from build123d import *

# Parameters (mm, degrees)
F0_R     = 50
F0_W     = 40
F0_H     = 40
F1_DEPTH = 25
F2_R     = 5
F3_SIZE2 = 5
F3_SIZE  = 2.3315382908


with BuildPart() as f1:
    # F0 (on Top) → F1 (new body)
    with BuildSketch(Plane.XY):
        Circle(F0_R)
        with Locations((0, -3.4369069617)):
            Rectangle(F0_W, F0_H, mode=Mode.SUBTRACT)
    extrude(amount=F1_DEPTH)

    # F2
    f2_edges = [f1.edges().sort_by_distance(p)[0] for p in [
        (0, 16.563093, 25),
        (-20, -3.436907, 25),
        (20, -3.436907, 25),
        (0, -23.436907, 25),
    ]]
    fillet(f2_edges, radius=F2_R)

    # F3
    f3_edges = [f1.edges().sort_by_distance(p)[0] for p in [
        (0, -23.436907, 0),
        (-20, -3.436907, 0),
        (0, 16.563093, 0),
        (20, -3.436907, 0),
    ]]
    f3_side = f1.faces().sort_by_distance((-48.585786, 0, 0))[0]
    chamfer(f3_edges, length=F3_SIZE, length2=F3_SIZE2, reference=f3_side)


solid = f1.part
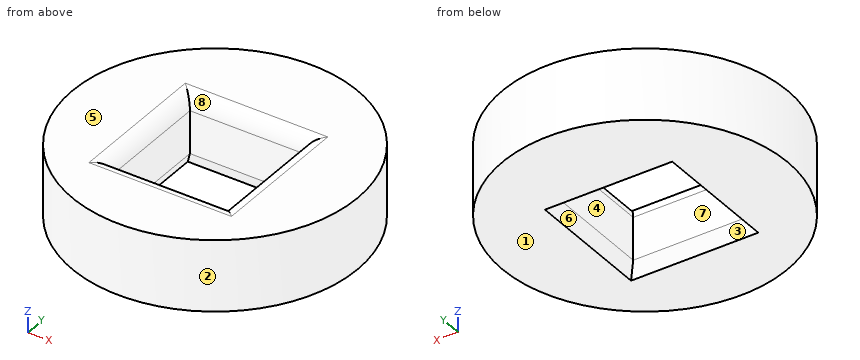
Design review of the part built by this model. Coordinates are the model's own, in mm. Face numbers are marked on the shaded views. A direction names the side the tool comes from. Round coordinates to 2 decimals unless told otherwise and drop trailing zeros. Loops run counter-clockwise (first coordinate to the right, second up) from the corner with the lowest first, then second, coordinate; pieces in that order, holes last. Notation, with made-up numbers: (56.5, 9) - (83.5, 9) arc R10 cw to (83.5, 14) - close; hole circle Ø10 at (52.5, -22). An arc over 180 degrees is marked (long way). One line per question, with ' | ' between items.
1. We need section A-A, the plane x = 0. State the section outline as (y, z) points, and give its area (3 significant figures).
Results are:
outline: (-50, 0) - (-25.77, 0) - (-23.44, 5) - (-23.44, 20) arc R5 ccw to (-28.44, 25) - (-50, 25) - close; (16.56, 5) - (18.89, 0) - (50, 0) - (50, 25) - (21.56, 25) arc R5 ccw to (16.56, 20) - close | area: 1,480 mm²
2. For L1, parallel to Y at x = -10, z = 15; L2, parallel to X at y = -1.5, z = 8.5; L3, parallel to Y at x = 2, z = 16.75, list the stretches that pass through material, from the lowest coordinate up. Write a range as [from, to].
Results are:
L1: y = [-48.99, -23.44], [16.56, 48.99] | L2: x = [-49.98, -20], [20, 49.98] | L3: y = [-49.96, -23.44], [16.56, 49.96]
3. Clearance check with flat-ended pins moving along their axes: P1, Ø1.5, axis at x = 30, z = 17.5, coming from the -Y side; P2, Ø7.5, axis at y = -9, z = 13.5, coming from the -X side; P3, Ø2, axis at x = -29, z = 18.5, coming from the +Y side. State where each tip first meets the part, or that it passes through.
Results are:
P1: stops at y = -40.55 | P2: stops at x = -49.72 | P3: stops at y = 41.42
4. We need section D-D, the plane z = 3.75. State the section outline as (x, y) points.
Results are:
outline: circle Ø100 at (0, 0); hole (-20.58, -24.02) - (20.58, -24.02) - (20.58, 17.15) - (-20.58, 17.15) - close
5. For the marked faces 5, 6, 7 and 8, list the 3-axis set-ups (+Z, -Z, +X, -X, +Y, -Y) from which the entire face can be reached by the end or side of a thin tool; tool diameter is ignored.
Results are:
face 5: +Z, +X, -X, +Y, -Y | face 6: -Z | face 7: +Z, -Z | face 8: +Z
6. We need section B-B, the plane y = -9. State the section outline as (x, z) points.
Results are:
outline: (-49.18, 0) - (-22.33, 0) - (-20, 5) - (-20, 20) arc R5 ccw to (-25, 25) - (-49.18, 25) - close; (20, 5) - (22.33, 0) - (49.18, 0) - (49.18, 25) - (25, 25) arc R5 ccw to (20, 20) - close
7. Draft analysis for pull direction Y (two halves, no side actions). For the marked faces 1, 2, 3 and 4, state which applies: released by +Y, released by -Y, zero draft, split by the parting line, or undercut.
Results are:
face 1: zero draft | face 2: split by the parting line | face 3: undercut | face 4: undercut
8. We need section C-C, the plane z = 15. State the section outline as (x, y) points.
Results are:
outline: circle Ø100 at (0, 0); hole (-20, -23.44) - (20, -23.44) - (20, 16.56) - (-20, 16.56) - close
